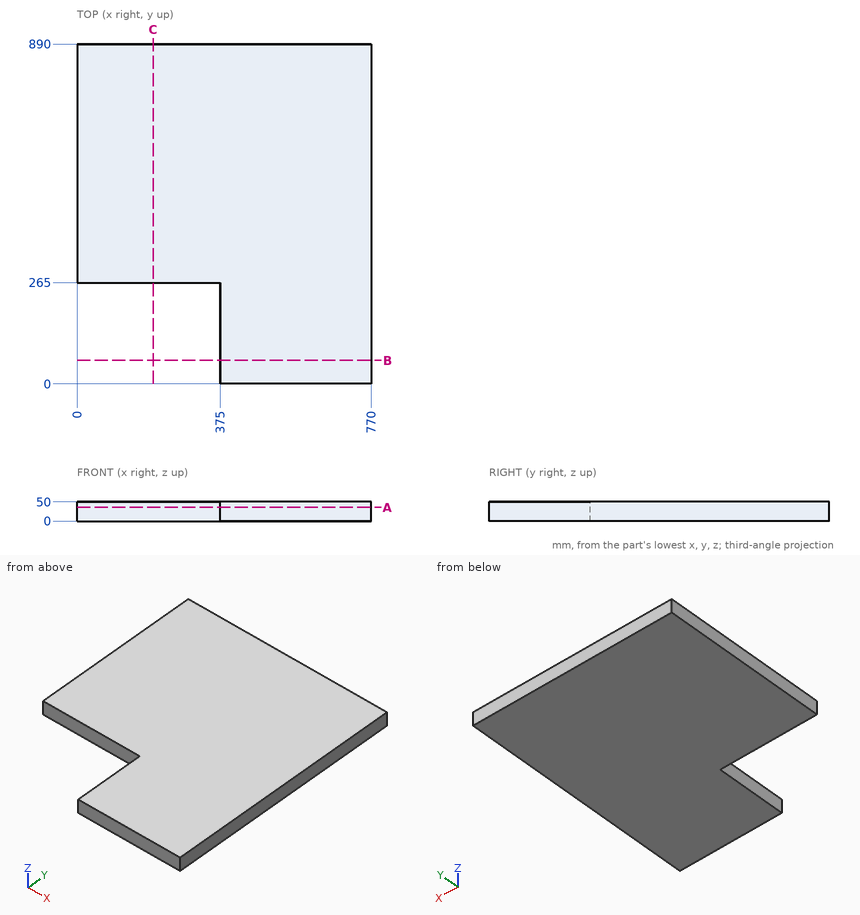
Answer from the drawing. Dimensions are ordinates in mm from the lowest x, y and z of the part. Coordinates: 2 decimals unless noted, no trailing zeros. Loops run counter-clockwise (first coordinate to the right, second up) from the corner with the lowest first, then second, coordinate; pieces in that order, holes last.
1) Section C-C (x = 199.5) is taken. Give the vertices of the cut face in (y, z).
Results:
outline: (265, 0) - (890, 0) - (890, 50) - (265, 50) - close
2) Section B-B (y = 61.5) is taken. Give the vertices of the cut face in (x, z), plus the area to 4 significant figures.
Results:
outline: (375, 0) - (770, 0) - (770, 50) - (375, 50) - close
area: 19,750 mm2
3) Consider probe 1 along Y at (x, z) = (174, 25); probe 2 along X at (y, z) = (81, 44). Determine where each line is inside the solid, lowest interval first.
Results:
probe 1: y = 265 to 890
probe 2: x = 375 to 770
4) Flat-ended cylindrical pins translate along their axes: pin 1 (25 mm diameter, centred on y = 111.5, z = 21.5, fed in from -X); pin 2 (6 mm diameter, centred on x = 362.5, y = 428.5, fed in from -Z); pin 3 (8 mm diameter, centred on x = 95.5, z = 8.5, fed in from -Y). Find the tip coordinate at first contact, or state that the pin passes through.
Results:
pin 1: stops at x = 375
pin 2: stops at z = 0
pin 3: stops at y = 265
5) Section A-A (z = 36) is taken. Give the vertices of the cut face in (x, y), plus the area to 3 significant figures.
Results:
outline: (0, 265) - (375, 265) - (375, 0) - (770, 0) - (770, 890) - (0, 890) - close
area: 586,000 mm2
